Part model, mm, in its own coordinate system. Face numbers are marked on the shaded views. Give positions to 0.01 mm unless a question says otherwise; leave off trailing zeros. Order: outer loops, then holes, each group sorted by start corner. A loop starts at its lowest first (then second) coordinate and runs counter-clockwise, first axis right, second up. Notation, with made-up numbers: (27, 48.5) - (77, 48.5) arc R23 ccw to (77, 78.5) - close; hole circle Ø9 at (-33, 44). An arc over 180 degrees is marked (long way). Use a Markdown table: item, result. Add a question column.
from build123d import *

# Parameters (mm, degrees)
SKETCH1_W           = 34
SKETCH1_H           = 30
SKETCH1_R           = 5.25
BOSS_EXTRUDE1_DEPTH = 30
SKETCH2_R           = 1.25
CUT_EXTRUDE1_DEPTH  = 10
SKETCH3_R           = 1.55
CUT_EXTRUDE2_DEPTH  = 10


with BuildPart() as part:
    # Sketch1 → Boss-Extrude1 (new body)
    with BuildSketch(Plane(origin=(0, 0, 0), x_dir=(1, 0, 0), z_dir=(0, 1, 0))):
        with Locations((17, -15)):
            Rectangle(SKETCH1_W, SKETCH1_H)
        with Locations(Location((17, -15, 0), (0, 0, 270))):
            Circle(SKETCH1_R, mode=Mode.SUBTRACT)
    extrude(amount=BOSS_EXTRUDE1_DEPTH)

    # Sketch2 → Cut-Extrude1 (cut)
    with BuildSketch(Plane.XZ):
        with Locations(Location((17, 23, 0), (0, 0, 270))):
            Circle(SKETCH2_R)
        with Locations(Location((25, 15, 0), (0, 0, 270))):
            Circle(SKETCH2_R)
        with Locations(Location((17, 7, 0), (0, 0, 270))):
            Circle(SKETCH2_R)
        with Locations(Location((9, 15, 0), (0, 0, 270))):
            Circle(SKETCH2_R)
    extrude(amount=-CUT_EXTRUDE1_DEPTH, mode=Mode.SUBTRACT)

    # Sketch3 → Cut-Extrude2 (cut)
    with BuildSketch(Plane.XY.offset(30)):
        with Locations((5, 25)):
            Circle(SKETCH3_R)
        with Locations((29, 25)):
            Circle(SKETCH3_R)
        with Locations((29, 5)):
            Circle(SKETCH3_R)
        with Locations((5, 5)):
            Circle(SKETCH3_R)
    extrude(amount=-CUT_EXTRUDE2_DEPTH, mode=Mode.SUBTRACT)


solid = part.part
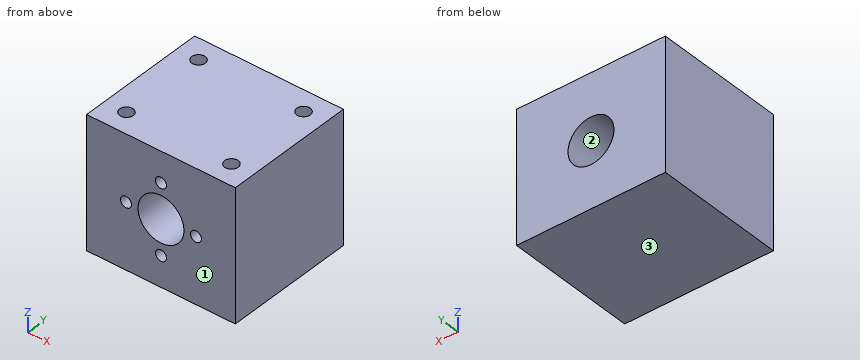
1. Drill centre lines: probe 1 along X at (y, z) = (7.25, 15); probe 2 along Y at (x, z) = (29, 22.5); probe 3 along X at (y, z) = (25.75, 24.25). Where is each one in solid material? Low to high. Write a range as [from, to].
2. Pin check, flat tips, straight feed: P1, Ø3, axis at x = 17, z = 7, coming from the -Y side; P2, Ø2, axis at x = 9, z = 15, coming from the -Y side; P3, Ø0.9, axis at x = 5.5, y = 24.5, coming from the +Z side. Stop position of each tip, or through.
3. Cut at A-A (y = 25). Write the cut outline in (x, z).
4. Cut at D-D (y = 5). Write the cut outline in (x, z), plus the area to 3 significant figures.
5. Cut at C-C (x = 25). Write the cut outline in (y, z), plus the area to 3 significant figures.
6. Cut at B-B (z = 26.5). Write the cut outline in (x, y), plus the area to 3 significant figures.
7. Mould opens along Z. For the marked faces 1, 2 and 3 say: released by +Z, released by -Z, zero draft, split by the parting line, or undercut.
Responses:
| question | item | result |
|---|---|---|
| 1 | probe 1 | x = [0, 7.75], [10.25, 11.75], [22.25, 23.75], [26.25, 34] |
| 1 | probe 2 | y = [0, 3.45], [6.55, 23.45], [26.55, 30] |
| 1 | probe 3 | x = [0, 3.64], [6.36, 27.64], [30.36, 34] |
| 2 | P1 | stops at y = 0 |
| 2 | P2 | stops at y = 10 |
| 2 | P3 | stops at z = 20 |
| 3 | outline | (0, 0) - (34, 0) - (34, 30) - (30.55, 30) - (30.55, 20) - (27.45, 20) - (27.45, 30) - (6.55, 30) - (6.55, 20) - (3.45, 20) - (3.45, 30) - (0, 30) - close; hole circle Ø10.5 at (17, 15) |
| 4 | outline | (0, 0) - (34, 0) - (34, 30) - (30.55, 30) - (30.55, 20) - (27.45, 20) - (27.45, 30) - (6.55, 30) - (6.55, 20) - (3.45, 20) - (3.45, 30) - (0, 30) - close; hole circle Ø2.5 at (9, 15); hole circle Ø10.5 at (17, 15); hole circle Ø2.5 at (17, 7); hole circle Ø2.5 at (17, 23); hole circle Ø2.5 at (25, 15) |
| 4 | area | 852 mm² |
| 5 | outline | (0, 0) - (30, 0) - (30, 30) - (0, 30) - (0, 16.25) - (10, 16.25) - (10, 13.75) - (0, 13.75) - close |
| 5 | area | 875 mm² |
| 6 | outline | (0, 0) - (34, 0) - (34, 30) - (0, 30) - close; hole circle Ø3.1 at (5, 5); hole circle Ø3.1 at (5, 25); hole circle Ø3.1 at (29, 5); hole circle Ø3.1 at (29, 25) |
| 6 | area | 990 mm² |
| 7 | face 1 | zero draft |
| 7 | face 2 | undercut |
| 7 | face 3 | released by -Z |
